Build history of the part. All positions in model axes, mm. A direction names the side the tool comes from. Round coordinates to 2 decimals unless told otherwise and drop trailing zeros. Order: outer loops, then holes, each group sorted by start corner. A loop starts at its lowest first (then second) coordinate and runs counter-clockwise, first axis right, second up. Notation, with made-up numbers: (-8, 45.5) -> (49, 45.5) arc R23 ccw to (49, 70.5) -> close; hole circle Ø4 at (65, -15.75). An arc over 180 degrees is marked (long way). Use a Markdown table: item, result. Add a question column.
Item 1: Slice it at A-A, the plane z = -6.5. Give the cut face in (x, y), plus the area to 3 significant figures.
Item 2: Slice it at D-D, the plane y = 6. Give the cut face in (x, z).
Item 3: Slice it at B-B, the plane x = 44.15. Give the cut face in (y, z).
Item 4: Probe L1, parallel to Z at x = 44, y = 20; L2, parallel to X at y = 18, z = -4; L3, parallel to X at y = 28, z = -7.5. List the from-to ranges inside material, lowest first.
Item 5: Slice it at C-C, the plane y = 21.5. Give the cut face in (x, z), plus the area to 3 significant figures.
Item 6: 3-axis set-ups, long thin cutter, end or side, ignore diameter. For faces 4 (the face through (40, 16, -6)), 5 (the face through (-40, 29, -6)), 6 (the face through (-40, 16, -6)), 7 (the face through (0.605, 27.493, -6.409)), 8 (the face through (40, 29, -6)): which of +Z, -Z, +X, -X, +Y, -Y reach the whole face in a straight line?
Item 7: Two-plate mould, pull along X, no slides. Class faces 1 (the face through (-31.2, 8, -6)), 2 (the face through (1, 28, 0)), 3 (the face through (47.845, 22.591, -4.968)): released by +X, released by -X, zero draft, split by the parting line, or undercut.
Item 8: Pin check, flat tips, straight feed: pin 1 (6.5 mm diameter, centred on x = 48, z = -5, fed in from +Y); pin 2 (2 mm diameter, centred on x = 9, z = -6.5, fed in from -Y); pin 3 (6 mm diameter, centred on x = -25.5, z = -10, fed in from -Y); pin 4 (6.5 mm diameter, centred on x = 40.5, z = -4, fed in from -Y). Stop position of each tip, or through.
from build123d import *

# Parameters (mm, degrees)
BOSS_EXTRUDE1_DEPTH = 13
SKETCH3_R           = 4
CUT_EXTRUDE1_DEPTH  = 13


with BuildPart() as part:
    # Sketch1 → Boss-Extrude1 (new body)
    with BuildSketch(Plane.XY):
        with BuildLine():
            Line((-27.5, 0), (-31.2, 0))
            Line((-31.2, 0), (-31.2, 16))
            Line((-31.2, 16), (-53.65, 16))
            Line((-53.65, 16), (-53.65, 29))
            Line((-53.65, 29), (-34.409301068, 29))
            ThreePointArc((-34.409301068, 29), (0, 45), (34.409301068, 29))
            Line((34.409301068, 29), (53.65, 29))
            Line((53.65, 29), (53.65, 16))
            Line((53.65, 16), (31.2, 16))
            Line((31.2, 16), (31.2, 0))
            Line((31.2, 0), (27.5, 0))
            ThreePointArc((27.5, 0), (0, 27.5), (-27.5, 0))
        make_face()
    extrude(amount=-BOSS_EXTRUDE1_DEPTH)

    # Sketch3 → Cut-Extrude1 (cut)
    with BuildSketch(Plane(origin=(0, 29, 0), x_dir=(1, 0, 0), z_dir=(0, 1, 0))):
        with Locations(Location((-44.15, 6.5, 0), (0, 0, 180))):
            Circle(SKETCH3_R)
        with Locations((44.15, 6.5)):
            Circle(SKETCH3_R)
    extrude(amount=-CUT_EXTRUDE1_DEPTH, mode=Mode.SUBTRACT)


solid = part.part
Check sheet entries:
| question | item | result |
|---|---|---|
| 1 | outline | (-53.65, 16) -> (-48.15, 16) -> (-48.15, 29) -> (-53.65, 29) -> close; (-40.15, 16) -> (-31.2, 16) -> (-31.2, 0) -> (-27.5, 0) arc R27.5 cw to (27.5, 0) -> (31.2, 0) -> (31.2, 16) -> (40.15, 16) -> (40.15, 29) -> (34.41, 29) arc R45 ccw to (-34.41, 29) -> (-40.15, 29) -> close; (48.15, 16) -> (53.65, 16) -> (53.65, 29) -> (48.15, 29) -> close |
| 1 | area | 1,760 mm2 |
| 2 | outline | (-31.2, -13) -> (-26.84, -13) -> (-26.84, 0) -> (-31.2, 0) -> close; (26.84, -13) -> (31.2, -13) -> (31.2, 0) -> (26.84, 0) -> close |
| 3 | outline | (16, -13) -> (29, -13) -> (29, -10.5) -> (16, -10.5) -> close; (16, -2.5) -> (29, -2.5) -> (29, 0) -> (16, 0) -> close |
| 4 | L1 | -13 to -10.5, -2.5 to 0 |
| 4 | L2 | -53.65 to -47.27, -41.03 to -20.79, 20.79 to 41.03, 47.27 to 53.65 |
| 4 | L3 | -53.65 to -48.02, -40.28 to 40.28, 48.02 to 53.65 |
| 5 | outline | (-53.65, -13) -> (-17.15, -13) -> (-17.15, 0) -> (-53.65, 0) -> close; (17.15, -13) -> (53.65, -13) -> (53.65, 0) -> (17.15, 0) -> close; hole circle Ø8 at (-44.15, -6.5); hole circle Ø8 at (44.15, -6.5) |
| 5 | area | 849 mm2 |
| 6 | face 4 | +Z, -Z, +X, -Y |
| 6 | face 5 | +Z, -Z, -X, +Y |
| 6 | face 6 | +Z, -Z, -X, -Y |
| 6 | face 7 | +Z, -Z, -Y |
| 6 | face 8 | +Z, -Z, +X, +Y |
| 7 | face 1 | released by -X |
| 7 | face 2 | zero draft |
| 7 | face 3 | undercut |
| 8 | pin 1 | y = 29 |
| 8 | pin 2 | y = 25.62 |
| 8 | pin 3 | y = 0 |
| 8 | pin 4 | y = 16 |
